Work out the finished part from the listing and answer in its coordinate system (mm). A direction names the side the tool comes from. Coordinates: 2 decimals unless noted, no trailing zeros. Loops run counter-clockwise (first coordinate to the right, second up) from the corner with the lowest first, then second, coordinate; pieces in that order, holes last. Notation, with made-up numbers: (41.25, -34.75) - (81.25, -34.75) arc R20 cw to (81.25, 4.25) - close; hole circle Ø7 at (77.5, -37.5). An arc over 180 degrees is marked (long way). Write each question's results on one line, items separated by ' | '. Start each with the question number.
1. Find the intervals of material crossed by line 1 along X through (y, z) = (71, 330) (3 decimals); line 2 along X through (y, z) = (59.5, 330.2) (3 decimals); line 3 along Z through (x, y) = (142, 73), in increasing order. Write a range as [from, to].
2. Determine the mould class of faces 1 (the conical face through (98.984, 30.772, 359.585)), 2 (the conical face through (113.797, 30.819, 359.585)), 3 (the flat face through (106, 38.1, 368)), 4 (the flat face through (80, 39, 361.95)) for opening direction Y: released by +Y, released by -Y, zero draft, split by the parting line, or undercut.
3. Each of these flat-tipped pins is pushed along its axis until it touches: P1, Ø4.5, axis at x = 20.64, z = 330.2, coming from the +Y side; P2, Ø6, axis at x = 62.5, y = 51, coming from the +Z side; P3, Ø10, axis at y = 32, z = 371.5, coming from the +X side. Where does it stop, or does it pass through?
4. A cutting plane is placed at A-A on y = 43.5. Determine the outline of the cut face in (x, z) (3 decimals), then the cut area to 3 significant figures.
5. Which of the six approach directions +Z, -Z, +X, -X, +Y, -Y give full straight-line access (tool end or side, diameter ignored) to faces 5 (the flat face through (92.075, 28, 368)), 6 (the cylindrical face through (118.95, 31.19, 368.21)), 7 (the flat face through (107, 19.05, 368)), 8 (the flat face through (120.65, 29, 368))?
6. A cutting plane is placed at B-B on x = 48. Determine the outline of the cut face in (y, z), then the cut area to 3 significant figures.
Autodesk Inventor part; units mm, degrees
ref_plane "YZ Plane" through (0, 0, 0) normal (1, 0, 0) x (0, 1, 0)
ref_plane "XZ Plane" through (0, 0, 0) normal (0, 1, 0) x (-1, 0, 0)
ref_plane "XY Plane" through (0, 0, 0) normal (0, 0, 1) x (1, 0, 0)
sketch "Sketch1" plane through (0, 0, 0) normal (0, 0, 1) x (1, 0, 0)
  line L0 (9.525, 0) -> (152.4, 0)
  line L1 (161.925, 9.525) -> (161.925, 76.2)
  line L2 (161.925, 76.2) -> (0, 76.2)
  line L3 (0, 76.2) -> (0, 9.525)
  line L4 (9.525, 0) -> (0, 9.525)
  line L5 (161.925, 9.525) -> (152.4, 0)
  point P0 (0, 0)
  point P1 (161.925, 0)
  dimension "d0" = 161.925
  dimension "d1" = 76.2
  dimension "d2" = 9.525
  dimension "d3" = 9.525
  dimension "d4" = 9.525
  dimension "d5" = 9.525
extrude "Main Body" add sketch "Sketch1" along normal blind 361.95
sketch "Sketch2" plane through (0, 0, 361.95) normal (0, 0, 1) x (1, 0, 0)
  line L0 (161.925, 76.2) -> (161.925, 9.525)
  line L1 (152.4, 0) -> (9.525, 0)
  line L2 (92.075, 38.1) -> (120.65, 38.1)
  line L3 (120.65, 38.1) -> (120.65, 19.05)
  line L4 (120.65, 19.05) -> (92.075, 19.05)
  line L5 (92.075, 19.05) -> (92.075, 38.1)
  point P0 (0, 0)
  dimension "d8" = 41.275
  dimension "d9" = 19.05
  dimension "d10" = 28.575
  dimension "d11" = 19.05
extrude "Terminal Block" add sketch "Sketch2" along normal blind 12.7
sketch "Sketch3" plane through (0, 0, 374.65) normal (0, 0, 1) x (1, 0, 0)
  line L0 (92.075, 38.1) -> (120.65, 38.1)
  line L1 (98.425, 30.1625) -> (114.3, 30.1625)
  point P0 (0, 0)
  point P1 (106.3625, 30.1625)
  point P2 (106.3625, 38.1)
  dimension "d14" = 15.875
  dimension "d15" = 7.9375
hole "Terminal Holes" at (98.425, 30.1625, 374.65) at (114.3, 30.1625, 374.65) direction (0, 0, -1) diameter 9.525 depth 12.7 tip angle 118
sketch "Sketch4" plane through (0, 76.2, 0) normal (0, 1, 0) x (1, 0, 0)
  line L0 (0, 0) -> (161.925, 0)
  line L1 (0, 0) -> (0, -361.95)
  line L2 (20.6375, -31.75) -> (141.2875, -31.75)
  line L3 (141.2875, -31.75) -> (141.2875, -330.2)
  line L4 (141.2875, -330.2) -> (20.6375, -330.2)
  line L5 (20.6375, -330.2) -> (20.6375, -31.75)
  point P0 (20.6375, -180.975)
  point P1 (0, -180.975)
  point P2 (80.9625, 0)
  point P3 (80.9625, -31.75)
  dimension "d23" = 120.65
  dimension "d24" = 298.45
hole "Hole2" at (20.6375, 76.2, 31.75) at (141.2875, 76.2, 31.75) at (141.2875, 76.2, 330.2) at (20.6375, 76.2, 330.2) direction (0, -1, 0) diameter 4.9784 depth 25.4 tip angle 118
properties part number "inverter"
Values:
1) line 1: [0, 18.156], [23.119, 138.806], [143.769, 161.925] | line 2: [0, 18.148], [23.127, 138.798], [143.777, 161.925] | line 3: [0, 29.36], [34.14, 327.81], [332.59, 361.95]
2) face 1: undercut | face 2: undercut | face 3: released by +Y | face 4: zero draft
3) P1: y = 50.66 | P2: z = 361.95 | P3: x = 120.65
4) outline: (0, 0) - (161.925, 0) - (161.925, 361.95) - (0, 361.95) - close | area: 58,600 mm^2
5) face 5: +Z, -X, +Y, -Y | face 6: +Z | face 7: +Z, +X, -X, -Y | face 8: +Z, +X, +Y, -Y
6) outline: (0, 0) - (76.2, 0) - (76.2, 361.95) - (0, 361.95) - close | area: 27,600 mm^2
